Study the drawing (mm; zero at the part's minimum x, y, z) and answer. A direction names the side the tool comes from. Give positions to 0.01 mm unless a question says otherwise; leave off trailing zeros. Write each loop counter-clockwise with the first axis right and the second up, starting at its lowest first coordinate (ties: lowest second). Pieces come first, ordered by that corner, then holes. Notation, with made-up numbers: (83, -21.75) - (91, -21.75) arc R26 ccw to (91, 6.25) - close; hole circle Ø9 at (54.5, -24.5). An arc over 180 degrees is marked (long way). Write each question's results on one line, items separated by ' | '. Start each with the question number.
Q1. For the marked faces 1 and 2, determine the directions among +Z, -Z, +X, -X, +Y, -Y from which every point of the face is accessible in a straight line to the end or side of a thin tool.
Q2. For a pull along Z with two mould halves and no side action, classify the marked faces 3, 4, 5 and 6 as pulls with the +Z half, pulls with the -Z half, needs draft (parallel to the pull), parting line crosses it, or undercut.
Q3. Section A-A (y = 19) is taken. Determine the outline of the cut face in (x, z), plus the area to 3 significant figures.
Q4. Find the intervals of material crossed by probe 1 along Z at (x, y) = (9, 34.5); probe 2 along Y at (x, z) = (39, 140), in increasing order.
Q5. A flat-ended cylindrical pin translates along its axis: pin 1 Ø12.5 at (x, z) = (28, 216) entering from -Y. Find the tip coordinate at first contact, or state that the pin passes through.
Q6. Section B-B (x = 45) is taken. Determine the outline of the cut face in (y, z), plus the area to 3 significant figures.
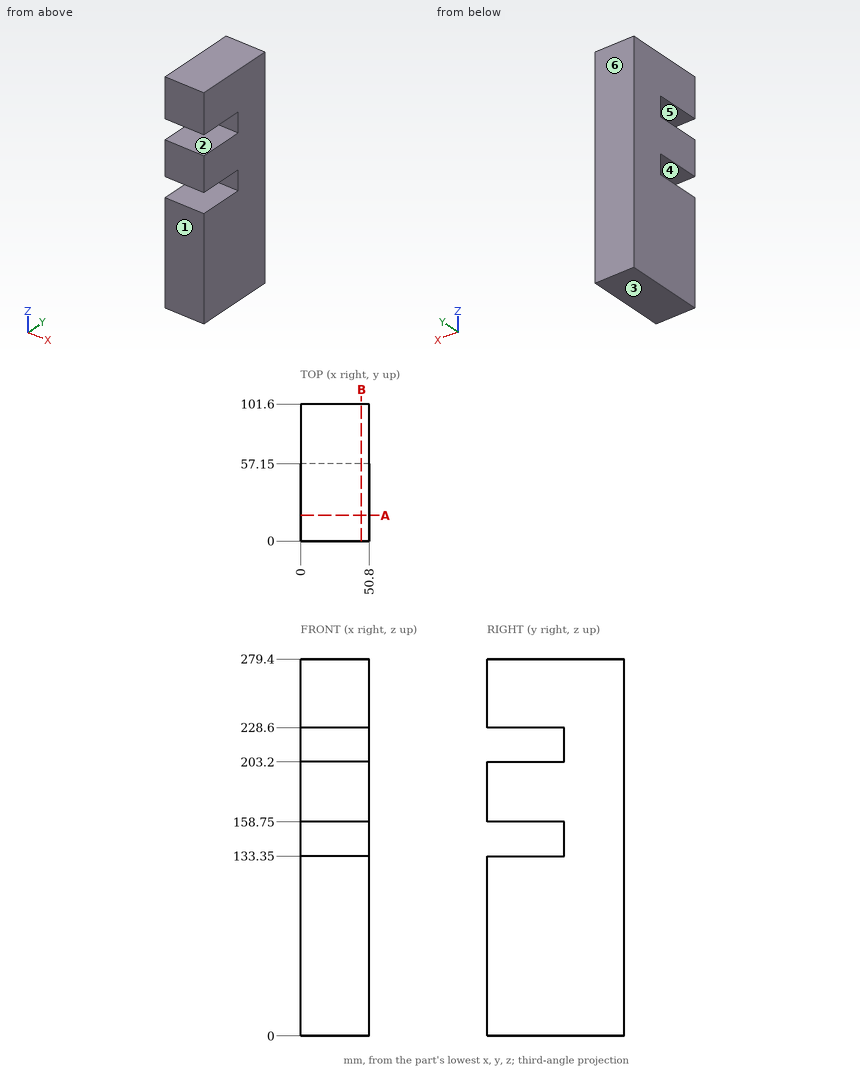
Answers below:
1) face 1: +Z, -Z, +X, -X, -Y | face 2: +X, -X, -Y
2) face 3: pulls with the -Z half | face 4: undercut | face 5: undercut | face 6: needs draft
3) outline: (0, 0) - (50.8, 0) - (50.8, 133.35) - (0, 133.35) - close; (0, 158.75) - (50.8, 158.75) - (50.8, 203.2) - (0, 203.2) - close; (0, 228.6) - (50.8, 228.6) - (50.8, 279.4) - (0, 279.4) - close | area: 11,600 mm2
4) probe 1: z = 0 to 133.35, 158.75 to 203.2, 228.6 to 279.4 | probe 2: y = 57.15 to 101.6
5) pin 1: stops at y = 57.15
6) outline: (0, 0) - (101.6, 0) - (101.6, 279.4) - (0, 279.4) - (0, 228.6) - (57.15, 228.6) - (57.15, 203.2) - (0, 203.2) - (0, 158.75) - (57.15, 158.75) - (57.15, 133.35) - (0, 133.35) - close | area: 25,500 mm2
